Input: part model. Units: mm. Frame: model coordinates. A direction names the side the tool comes from. Give positions to 0.01 mm unless a question says otherwise; leave off trailing zeros. Loops run counter-clockwise (first coordinate to the right, second up) from the corner with the lowest first, then second, coordinate; pieces in that order, holes last.
Autodesk Inventor part; units mm, degrees
ref_plane "YZ Plane" through (0, 0, 0) normal (1, 0, 0) x (0, 1, 0)
ref_plane "XZ Plane" through (0, 0, 0) normal (0, 1, 0) x (-1, 0, 0)
ref_plane "XY Plane" through (0, 0, 0) normal (0, 0, 1) x (1, 0, 0)
sketch "Sketch1" plane through (0, 0, 0) normal (0, 1, 0) x (-1, 0, 0)
  line L0 (374.65, 374.65) -> (-374.65, 374.65)
  line L1 (-374.65, 374.65) -> (-374.65, -374.65)
  line L2 (-374.65, -374.65) -> (374.65, -374.65)
  line L3 (374.65, -374.65) -> (374.65, 374.65)
  line L4 (374.65, 374.65) -> (-374.65, -374.65) construction
  line L5 (-374.65, 374.65) -> (374.65, -374.65) construction
  line L6 (457.2, 457.2) -> (-457.2, 457.2)
  line L7 (-457.2, 457.2) -> (-457.2, -457.2)
  line L8 (-457.2, -457.2) -> (457.2, -457.2)
  line L9 (457.2, -457.2) -> (457.2, 457.2)
  line L10 (457.2, 457.2) -> (-457.2, -457.2) construction
  line L11 (-457.2, 457.2) -> (457.2, -457.2) construction
  point P0 (0, 0)
  dimension "d0" = 82.55
  dimension "d1" = 82.55
  dimension "d2" = 749.3
  dimension "d3" = 749.3
extrude "Extrusion1" add sketch "Sketch1" along normal blind 127
fillet "Fillet1" radius 31.75 12 edges at (0, 127, 457.2) (0, 0, 457.2) (457.2, 63.5, 457.2) (457.2, 127, 0) (457.2, 0, 0) (457.2, 63.5, -457.2) (0, 127, -457.2) (-457.2, 127, 0) (-457.2, 63.5, 457.2) (0, 0, -457.2) (-457.2, 63.5, -457.2) (-457.2, 0, 0)
sketch "Bumper_Gaps" plane through (0, 127, 0) normal (0, 1, 0) x (1, 0, 0)
  line L0 (-222.25, -457.2) -> (222.25, -457.2)
  line L1 (222.25, -457.2) -> (222.25, -374.65)
  line L2 (222.25, -374.65) -> (-222.25, -374.65)
  line L3 (-222.25, -374.65) -> (-222.25, -457.2)
  line L4 (-222.25, -457.2) -> (222.25, -374.65) construction
  line L5 (222.25, -457.2) -> (-222.25, -374.65) construction
  line L6 (-457.2, -254) -> (-374.65, -254)
  line L7 (-374.65, -254) -> (-374.65, 254)
  line L8 (-374.65, 254) -> (-457.2, 254)
  line L9 (-457.2, 254) -> (-457.2, -254)
  line L10 (-457.2, -254) -> (-374.65, 254) construction
  line L11 (-374.65, -254) -> (-457.2, 254) construction
  line L12 (374.65, -254) -> (457.2, -254)
  line L13 (457.2, -254) -> (457.2, 254)
  line L14 (457.2, 254) -> (374.65, 254)
  line L15 (374.65, 254) -> (374.65, -254)
  line L16 (374.65, -254) -> (457.2, 254) construction
  line L17 (457.2, -254) -> (374.65, 254) construction
  line L18 (-374.65, -374.65) -> (-374.65, 374.65)
  line L19 (-457.2, 425.45) -> (-457.2, -425.45)
  line L20 (374.65, 374.65) -> (374.65, -374.65)
  line L21 (457.2, -425.45) -> (457.2, 425.45)
  line L22 (374.65, -374.65) -> (-374.65, -374.65)
  line L23 (-425.45, -457.2) -> (425.45, -457.2)
  line L24 (-196.85, 374.65) -> (196.85, 374.65)
  line L25 (196.85, 374.65) -> (196.85, 457.2)
  line L26 (196.85, 457.2) -> (-196.85, 457.2)
  line L27 (-196.85, 457.2) -> (-196.85, 374.65)
  line L28 (-196.85, 374.65) -> (196.85, 457.2) construction
  line L29 (196.85, 374.65) -> (-196.85, 457.2) construction
  line L30 (425.45, 457.2) -> (-425.45, 457.2)
  line L31 (-374.65, 374.65) -> (374.65, 374.65)
  point P0 (0, 0)
  point P1 (0, -415.925)
  point P2 (-415.925, 0)
  point P3 (415.925, 0)
  point P4 (0, 415.925)
  dimension "d15" = 444.5
  dimension "d16" = 393.7
  dimension "d17" = 508
  dimension "d18" = 508
extrude "Front_Gap" cut sketch "Bumper_Gaps" against normal through all contours L3 L2 L1 L0
extrude "Back_Gap" [suppressed]
extrude "Left_Gap" [suppressed]
extrude "Right_Gap" [suppressed]
equation "\"d1\" = d0"
equation "\"d2\" = Length"
equation "\"d3\" = Width"
equation "\"d15\" = Front_Width"
equation "\"d16\" = Back_Width"
equation "\"d17\" = Left_Width"
equation "\"d18\" = Right_Width"
equation "\"Length\" = 749.3"
equation "\"Width\" = 749.3"
equation "\"Front_Width\" = 444.5"
equation "\"Back_Width\" = 393.7"
equation "\"Left_Width\" = 508"
equation "\"Right_Width\" = 508"
equation "\"Front_Edge\" = 152.4"
equation "\"Back_Edge\" = 152.4"
equation "\"Left_Edge\" = 152.4"
equation "\"Right_Edge\" = 152.4"
equation "\"FECalc\" = -0.5 * Front_Width + 0.5 * Width"
equation "\"BECalc\" = -0.5 * Back_Width + 0.5 * Width"
equation "\"LECalc\" = -0.5 * Left_Width + 0.5 * Length"
equation "\"RECalc\" = -0.5 * Right_Width + 0.5 * Length"
equation "\"FWCalc\" = Width - 2 * Front_Edge"
equation "\"BWCalc\" = Width - 2 * Back_Edge"
equation "\"LWCalc\" = Length - 2 * Left_Edge"
equation "\"RWCalc\" = Length - 2 * Right_Edge"
properties part number "Bumper Template (WIP)"
(1) Cut plane B-B (x = -333). Return the cut outline in (y, z), and give its area (3 significant figures).
Values follow:
outline: (0, -425.45) arc R31.75 ccw to (31.75, -457.2) - (95.25, -457.2) arc R31.75 ccw to (127, -425.45) - (127, -374.65) - (0, -374.65) - close; (0, 374.65) - (127, 374.65) - (127, 425.45) arc R31.75 ccw to (95.25, 457.2) - (31.75, 457.2) arc R31.75 ccw to (0, 425.45) - close
area: 20,100 mm2
(2) Cut plane D-D (x = 150.5). Return the cut outline in (y, z).
Values follow:
outline: (0, -425.45) arc R31.75 ccw to (31.75, -457.2) - (95.25, -457.2) arc R31.75 ccw to (127, -425.45) - (127, -374.65) - (0, -374.65) - close
(3) Cut plane A-A (z = -108). Return the cut outline in (x, y), and give its area (3 significant figures).
Values follow:
outline: (-457.2, 31.75) arc R31.75 ccw to (-425.45, 0) - (-374.65, 0) - (-374.65, 127) - (-425.45, 127) arc R31.75 ccw to (-457.2, 95.25) - close; (374.65, 0) - (425.45, 0) arc R31.75 ccw to (457.2, 31.75) - (457.2, 95.25) arc R31.75 ccw to (425.45, 127) - (374.65, 127) - close
area: 20,100 mm2
(4) Cut plane C-C (y = 42.5). Return the cut outline in (x, z).
Values follow:
outline: (-457.2, -425.45) arc R31.75 ccw to (-425.45, -457.2) - (425.45, -457.2) arc R31.75 ccw to (457.2, -425.45) - (457.2, 425.45) arc R31.75 ccw to (425.45, 457.2) - (222.25, 457.2) - (222.25, 374.65) - (374.65, 374.65) - (374.65, -374.65) - (-374.65, -374.65) - (-374.65, 374.65) - (-222.25, 374.65) - (-222.25, 457.2) - (-425.45, 457.2) arc R31.75 ccw to (-457.2, 425.45) - close
(5) Reachability of faces 1 (the flat face through (2, 127, -408)), 2 (the flat face through (-374.65, 63, -5)) from +Z, -Z, +X, -X, +Y, -Y: full face, straight path, thin tool, end or side. Return the list, or none.
Values follow:
face 1: +Z, -Z, +X, -X, +Y
face 2: +Y, -Y
(6) Pin query (flat end, axial travel): pin 1 Ø1.5 at (x, y) = (-326, 23.5) entering from -Z. Return the tip coordinate at first contact, or that it passes through.
Values follow:
pin 1: stops at z = -456.3
(7) Ray query, probe 1 along X at (y, z) = (90.5, 97); probe 2 along Z at (x, y) = (71, 79). Return the intervals inside material, ascending.
Values follow:
probe 1: x = -457.2 to -374.65, 374.65 to 457.2
probe 2: z = -457.2 to -374.65
(8) Mould query, pull axis X, two halves, no side actions, for faces 3 (the flat face through (6, 63, -457.2)), 4 (the cylindrical face through (-447.7, 63.9, -448.1)), 5 (the cylindrical face through (447.7, 117.9, -6)), 6 (the flat face through (297, 63, 374.65)). Classes: +X half, -X half, draft (parallel to the pull), parting line (faces both ways), or undercut.
Values follow:
face 3: draft
face 4: -X half
face 5: +X half
face 6: undercut
